Can you work these out from the model? Positions are in its coordinate system, mm. Round coordinates to 2 decimals unless told otherwise and drop trailing zeros. Order: outer loops, then holes, each group sorted by start corner. A loop starts at its lowest first (then second) coordinate and runs counter-clockwise, first axis right, second up. Notation, with made-up numbers: M 49,-12.5 L 73,-12.5 A30 cw 73,26.5 Z; hole C 69.5,76 d1. An arc over 180 degrees is marked long. Answer as a JSON object with one key per item and string values. Group by question number.
Autodesk Inventor part; units mm, degrees
ref_plane "Arbeitsebene1" through (0, 0, 4) normal (0, 0, 1) x (1, 0, 0)
ref_plane "YZ Plane" through (0, 0, 0) normal (1, 0, 0) x (0, 1, 0)
ref_plane "XZ Plane" through (0, 0, 0) normal (0, 1, 0) x (-1, 0, 0)
sketch "Skizze1" plane through (0, 0, 0) normal (0, 0, 1) x (1, 0, 0)
  line L0 (0, -28) -> (0, 28)
  line L1 (-28, 0) -> (28, 0)
  circle A0 centre (0, 0) radius 20
  dimension "d0" = 40
extrude "Extrusion1" add sketch "Skizze1" along normal mid plane 10.4
ref_plane "Arbeitsebene1" through (0, 0, 4) normal (0, 0, 1) x (1, 0, 0)
sketch "Skizze3" plane through (0, 0, 4) normal (0, 0, 1) x (1, 0, 0)
  arc A0 (-5, 0) -> (5, 0) centre (0, 0) ccw
  line L0 (-28, 0) -> (28, 0)
  line L1 (-5, 0) -> (5, 0)
  dimension "d4" = 10
revolve "Umdrehung1" cut sketch "Skizze3" angle 360 about axis through (-10, 0, 4) along (1, 0, 0)
sketch "Skizze4" plane through (0, 0, 0) normal (0, 1, 0) x (-1, 0, 0)
  line L0 (-20, -5.2) -> (20, -5.2)
  line L1 (20, 5.2) -> (-20, 5.2)
  line L2 (-20, -5.2) -> (-20, 5.2)
  line L3 (28, 0) -> (-28, 0)
  line L4 (0, -7.28) -> (0, 7.28)
  line L5 (20, 5.2) -> (-20, 5.2)
  line L6 (-7.8, 5.2) -> (-20, -1.9841)
  line L7 (-20, -1.9841) -> (-20, 5.2)
  line L8 (-20, 5.2) -> (-7.8, 5.2)
  point P0 (0, 0)
revolve "Umdrehung2" cut sketch "Skizze4" angle 360 about axis through (0, 0, -10) along (0, 0, 1) contours L2 L3 L6 | L2 L1 L6 L3
properties part number "Plastikfuß_40mm" material "ABS-Kunststoff"
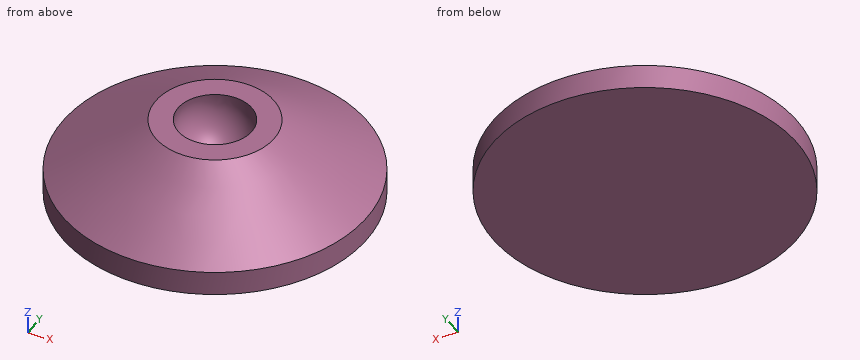
1) If we section it at A-A on x = 0: Write out the boundary of the cut face in (y, z).
2) For pin 1 (12 mm diameter, centred on x = -12, y = -9, fed in from +Z); pin 2 (4.5 mm diameter, centred on x = -3, y = -2, fed in from +Z); pin 3 (8 mm diameter, centred on y = -2.5, z = 6, fed in from +X), each with a flat end and sliding along its axis, tell me the tip position at first contact or that it passes through.
3) If we section it at B-B on z = 2.75: Write out the boundary of the cut face in (x, y), plus the area to 3 significant figures.
4) I need wall thicknesses on line 1 along X through (y, z) = (-1, 0); line 2 along Z through (x, y) = (-4, 6); line 3 along X through (y, z) = (0.5, 2.75). Which ranges of each line are inside material? Lowest first, please.
Findings:
{
 "1": {"outline": "M -20,-5.2 L 20,-5.2 L 20,-1.98 L 7.8,5.2 L 4.85,5.2 A5 cw long -4.85,5.2 L -7.8,5.2 L -20,-1.98 Z"},
 "2": {"pin 1": "stops at z = 4.49", "pin 2": "stops at z = 5.2", "pin 3": "stops at x = 13.03"},
 "3": {"outline": "C 0,0 d23.92; hole C 0,0 d9.68", "area": "376 mm^2"},
 "4": {"line 1": "x = -16.6 to -2.83, 2.83 to 16.6", "line 2": "z = -5.2 to 5.2", "line 3": "x = -11.95 to -4.82, 4.82 to 11.95"}
}
